```python
from build123d import *

# Parameters (mm, degrees)
SKETCH1_R           = 4.95
BOSS_EXTRUDE2_DEPTH = 6.6
SKETCH4_R           = 11.5
BOSS_EXTRUDE3_DEPTH = 1
SKETCH5_R           = 9
BOSS_EXTRUDE4_DEPTH = 12
SKETCH6_R           = 11.5
BOSS_EXTRUDE5_DEPTH = 1
FILLET1_R           = 1
FILLET2_R           = 1
SKETCH7_R           = 2.5
CUT_EXTRUDE1_DEPTH  = 21.6


with BuildPart() as part:
    # Sketch1 → Boss-Extrude2 (new body)
    with BuildSketch(Plane(origin=(0, 0, 0), x_dir=(1, 0, 0), z_dir=(0, 1, 0))):
        Circle(SKETCH1_R)
    extrude(amount=BOSS_EXTRUDE2_DEPTH)

    # Sketch4 → Boss-Extrude3 (add)
    with BuildSketch(Plane(origin=(0, 6.6, 0), x_dir=(1, 0, 0), z_dir=(0, 1, 0))):
        Circle(SKETCH4_R)
    extrude(amount=BOSS_EXTRUDE3_DEPTH)

    # Sketch5 → Boss-Extrude4 (add)
    with BuildSketch(Plane(origin=(0, 7.6, 0), x_dir=(1, 0, 0), z_dir=(0, 1, 0))):
        with Locations((0, 0.291114712)):
            Circle(SKETCH5_R)
    extrude(amount=BOSS_EXTRUDE4_DEPTH)

    # Sketch6 → Boss-Extrude5 (add)
    with BuildSketch(Plane(origin=(0, 19.6, 0), x_dir=(1, 0, 0), z_dir=(0, 1, 0))):
        Circle(SKETCH6_R)
    extrude(amount=BOSS_EXTRUDE5_DEPTH)

    # Fillet1
    fillet1_edges = [part.edges().sort_by_distance(p)[0] for p in [
        (-9, 7.6, -0.291114712),
    ]]
    fillet(fillet1_edges, radius=FILLET1_R)

    # Fillet2
    fillet2_edges = [part.edges().sort_by_distance(p)[0] for p in [
        (-9, 19.6, -0.291114712),
    ]]
    fillet(fillet2_edges, radius=FILLET2_R)

    # Sketch7 → Cut-Extrude1 (cut, through all)
    with BuildSketch(Plane.XZ):
        Circle(SKETCH7_R)
    extrude(amount=-CUT_EXTRUDE1_DEPTH, mode=Mode.SUBTRACT)


solid = part.part
```
Could you check a few things on this model? Use its own coordinates, in mm. A direction names the side the tool comes from. Coordinates: 2 decimals unless noted, no trailing zeros. Write each loop counter-clockwise with the first axis right and the second up, starting at its lowest first coordinate (ties: lowest second). Pieces come first, ordered by that corner, then holes. Notation, with made-up numbers: (-20.5, 1) - (38.5, 1) arc R23 ccw to (38.5, 37) - close; hole circle Ø11 at (-5.5, 52.25). An arc over 180 degrees is marked (long way). Use a Markdown table: item, result.
Q1. Imagine slicing it at A-A (x = 0). List the corners of the cut face in (y, z) for me, and give its area (3 significant figures).
Geometry check:
| item | result |
|---|---|
| outline | (0, -4.95) - (6.6, -4.95) - (6.6, -11.5) - (7.6, -11.5) - (7.6, -10.29) arc R1 cw to (8.6, -9.29) - (18.6, -9.29) arc R1 cw to (19.6, -10.29) - (19.6, -11.5) - (20.6, -11.5) - (20.6, -2.5) - (0, -2.5) - close; (0, 2.5) - (20.6, 2.5) - (20.6, 11.5) - (19.6, 11.5) - (19.6, 9.71) arc R1 cw to (18.6, 8.71) - (8.6, 8.71) arc R1 cw to (7.6, 9.71) - (7.6, 11.5) - (6.6, 11.5) - (6.6, 4.95) - (0, 4.95) - close |
| area | 225 mm2 |
Q2. I'm going to push flat-ended pins straight in: pin 1 Ø2 at (y, z) = (4.5, 4.5) entering from -X; pin 2 Ø5 at (x, y) = (0.5, 10) entering from -Z; pin 3 Ø3 at (x, z) = (-5.5, -3.5) entering from -Y; pin 4 Ø12 at (x, y) = (6, 12.5) entering from -Z. Where does each tip first touch, or does it pass through?
Geometry check:
| item | result |
|---|---|
| pin 1 | stops at x = -3.5 |
| pin 2 | stops at z = -11.5 |
| pin 3 | stops at y = 6.6 |
| pin 4 | stops at z = -11.22 |
Q3. Thinking about a two-plate mould opening in Y: for faces 1 (the flat face through (2, 0, 2)), 2 (the flat face through (5.1, 19.6, 8.5)), 3 (the cylindrical face through (-1.5, 20.1, -11.4)), which applies, +Y half, -Y half, draft (parallel to the pull), parting line (faces both ways), or undercut?
Geometry check:
| item | result |
|---|---|
| face 1 | -Y half |
| face 2 | undercut |
| face 3 | draft |
Q4. Imagine slicing it at B-B (y = 5). List the corners of the cut face in (x, z) for me, and give its area (3 significant figures).
Geometry check:
| item | result |
|---|---|
| outline | circle Ø9.9 at (0, 0); hole circle Ø5 at (0, 0) |
| area | 57.3 mm2 |
Q5. Imagine slicing it at C-C (y = 15). List the corners of the cut face in (x, z) for me, and give its area (3 significant figures).
Geometry check:
| item | result |
|---|---|
| outline | circle Ø18 at (0, -0.29); hole circle Ø5 at (0, 0) |
| area | 235 mm2 |
Q6. Please list where these lines run through material, in increasing order: L1, parallel to Y at x = 4, z = -9.5; L2, parallel to Z at x = 0, y = 11; L3, parallel to Y at x = 6.5, z = 1.5.
Geometry check:
| item | result |
|---|---|
| L1 | y = 6.6 to 7.6, 19.6 to 20.6 |
| L2 | z = -9.29 to -2.5, 2.5 to 8.71 |
| L3 | y = 6.6 to 20.6 |
Q7. Which directions (+Z, -Z, +X, -X, +Y, -Y) give clear straight access to the entire face, cutting with the end or side of a thin tool? Please do faces 4 (the cylindrical face through (-8.99, 13.53, -0.69)), 5 (the flat face through (5, 6.6, 2)), 6 (the cylindrical face through (-0.54, 10.16, -2.44)).
Geometry check:
| item | result |
|---|---|
| face 4 | none |
| face 5 | -Y |
| face 6 | +Y, -Y |
